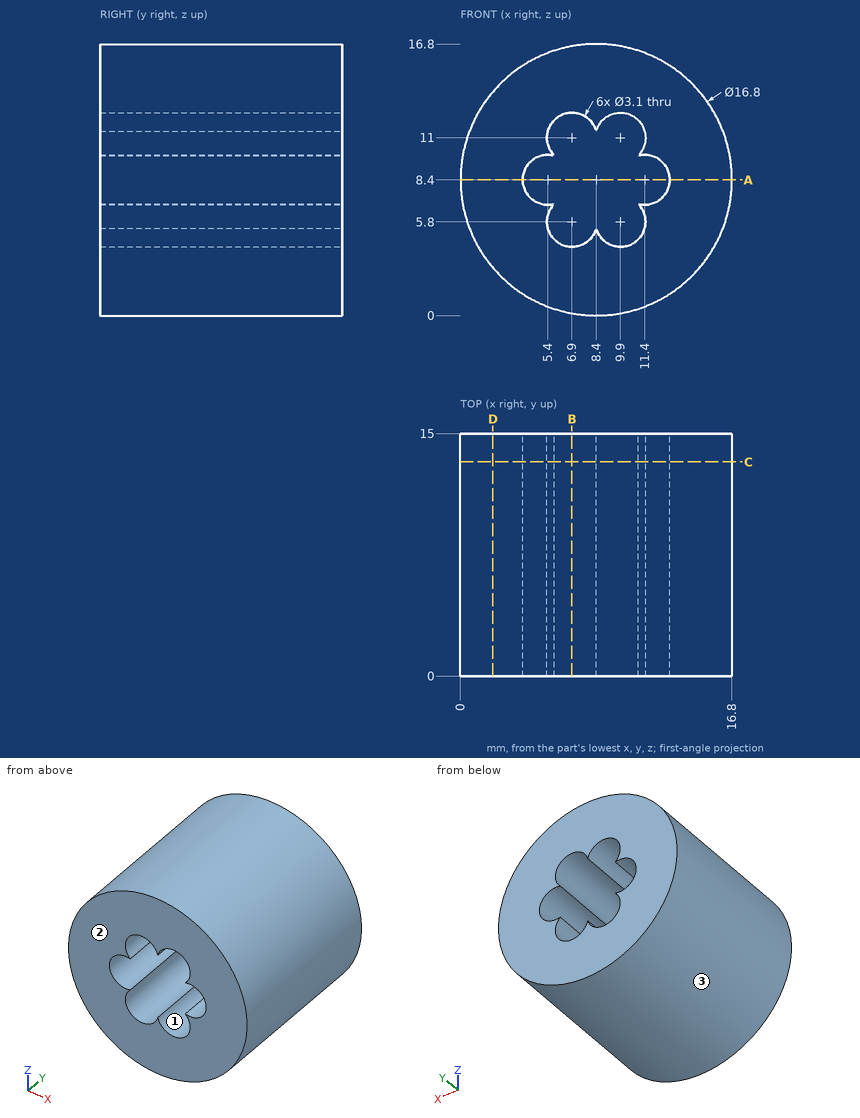
Geometry: see drawing. Coordinates: mm, zero at the bounding-box minimum. Round coordinates to 2 decimals unless told otherwise and drop trailing zeros. Write each loop counter-clockwise with the first axis right and the second up, starting at its lowest first coordinate (ties: lowest second). Pieces come first, ordered by that corner, then holes.
Item 1: Section query A-A (z = 8.4). Return loops of the section in (x, y), plus the area to 4 significant figures.
Item 2: Section query B-B (x = 6.9). Return loops of the section in (y, z).
Item 3: Material intervals for L1, parallel to Z at x = 5.5, y = 9.5; L2, parallel to X at y = 6.75, z = 10.5; L3, parallel to Z at x = 6.9, y = 4, sorted ascending.
Item 4: Pin query (flat end, axial travel): P1, Ø2, axis at x = 5, y = 3, coming from the -Z side; P2, Ø5, axis at y = 12.5, z = 4.5, coming from the +X side; P3, Ø3, axis at x = 5.4, z = 8.4, coming from the -Y side; P4, Ø3, axis at y = 13, z = 3, coming from the -X side. Return the tip coordinate at first contact, or that it passes through.
Item 5: Section query C-C (y = 13.25). Return loops of the section in (x, z).
Item 6: Mould query, pull axis X, two halves, no side actions, for the marked faces 1, 2 and 3. Classes: +X half, -X half, draft (parallel to the pull), parting line (faces both ways), or undercut.
Item 7: Section query D-D (x = 2). Return loops of the section in (y, z), plus the area to 3 significant figures.
Completed:
1. outline: (0, 0) - (3.85, 0) - (3.85, 15) - (0, 15) - close; (12.95, 0) - (16.8, 0) - (16.8, 15) - (12.95, 15) - close
1. area: 115.5 mm2
2. outline: (0, 0.14) - (15, 0.14) - (15, 4.25) - (0, 4.25) - close; (0, 12.55) - (15, 12.55) - (15, 16.66) - (0, 16.66) - close
3. L1: z = 0.52 to 5.13, 6.47 to 6.85, 9.95 to 10.33, 11.67 to 16.28
3. L2: x = 0.27 to 5.43, 11.37 to 16.53
3. L3: z = 0.14 to 4.25, 12.55 to 16.66
4. P1: stops at z = 0.35
4. P2: stops at x = 16.68
4. P3: passes through
4. P4: stops at x = 0.96
5. outline: circle Ø16.8 at (8.4, 8.4); hole (5.81, 6.91) arc R1.55 ccw (long way) to (8.4, 5.41) arc R1.55 ccw (long way) to (10.99, 6.91) arc R1.55 ccw (long way) to (10.99, 9.89) arc R1.55 ccw (long way) to (8.4, 11.39) arc R1.55 ccw (long way) to (5.81, 9.89) arc R1.55 ccw (long way) to start
6. face 1: undercut
6. face 2: draft
6. face 3: parting line
7. outline: (0, 2.96) - (15, 2.96) - (15, 13.84) - (0, 13.84) - close
7. area: 163 mm2
